```python
from build123d import *

# Parameters (mm, degrees)
BOSS_EXTRUDE1_DEPTH          = 19.05
SKETCH2_W                    = 12.7
SKETCH2_H                    = 9.652
CUT_EXTRUDE1_DEPTH           = 108.035088344
BOSS_EXTRUDE2_DEPTH          = 3.175
CUT_EXTRUDE12_DEPTH          = 7.9375
F_1_2_0_375_DIAMETER_HOLE1_D = 9.525
F_1_2_0_375_DIAMETER_HOLE2_D = 9.525


with BuildPart() as part:
    # Sketch1 → Boss-Extrude1 (new, symmetric)
    with BuildSketch(Plane.XY):
        with BuildLine():
            Line((0, 36.148070179), (0, 0))
            Line((0, 0), (88.9, 0))
            Line((88.9, 0), (88.9, 19.05))
            Line((88.9, 19.05), (28.593563708, 53.867937227))
            ThreePointArc((28.593563708, 53.867937227), (8.995572876, 53.562269727), (0, 36.148070179))
        make_face()
    extrude(amount=BOSS_EXTRUDE1_DEPTH, both=True)

    # Sketch2 → Cut-Extrude1 (cut, through all)
    with BuildSketch(Plane(origin=(88.9, 0, 0), x_dir=(0, 0, -1), z_dir=(1, 0, 0))):
        with Locations((0, 4.826)):
            Rectangle(SKETCH2_W, SKETCH2_H)
    extrude(amount=-CUT_EXTRUDE1_DEPTH, mode=Mode.SUBTRACT)

    # Sketch3 → Boss-Extrude2 (add, symmetric)
    with BuildSketch(Plane.XY.offset(12.7)):
        Polygon((88.9, 28.728699913), (61.669909488, 44.45), (44.905909488, 44.45), (88.9, 19.05), align=None)
    extrude(amount=BOSS_EXTRUDE2_DEPTH, both=True)

    # Sketch17 → Cut-Extrude12 (cut, symmetric)
    with BuildSketch(Plane.XY):
        Polygon((0, 25.4), (33.782, 25.4), (51.929375197, 56.832175865), (0, 56.832175865), align=None)
    extrude(amount=CUT_EXTRUDE12_DEPTH, both=True, mode=Mode.SUBTRACT)

    # 1/2 (0.375) Diameter Hole1 (through all)
    with Locations(Plane(origin=(30.473891971, 52.782329198, 0), x_dir=(0.8660254037844419, -0.4999999999999945, 0), z_dir=(0.49999999999999445, 0.8660254037844418, 0))):
        with Locations((42.064658396, 0)):
            Hole(F_1_2_0_375_DIAMETER_HOLE1_D / 2)

    # 1/2 (0.375) Diameter Hole2 (through all)
    with Locations(Plane.XY.offset(19.05)):
        with Locations((19.05, 37.338)):
            Hole(F_1_2_0_375_DIAMETER_HOLE2_D / 2)


solid = part.part
```
Source: CAD feature listing. Evaluate the final solid. Frame: model axes, mm. A direction names the side the tool comes from. Coordinates: 2 decimals unless noted, no trailing zeros. Write each loop counter-clockwise with the first axis right and the second up, starting at its lowest first coordinate (ties: lowest second). Pieces come first, ordered by that corner, then holes. Notation, with made-up numbers: (-27.5, -18) - (7.5, -18) arc R23 ccw to (7.5, 3) - close; hole circle Ø5 at (-3.75, 25.5). An arc over 180 degrees is marked (long way). Answer as a JSON object with one key per item and string values.
Q1. Set-up query: faces 4 (the cylindrical face through (16.49, 41.354, -13.572)), 5 (the flat face through (45, 5, -6.35)), 6 (the flat face through (53, 44.45, 13)), 7 (the flat face through (72, 35, 15.875)). Return all of +Z, -Z, +X, -X, +Y, -Y with unobstructed straight access to the full face (end or side cutting, diameter ignored); none if empty.
Ans:
{"face 4": "+Z, -Z", "face 5": "+X, -X, -Y", "face 6": "+Z, -Z, +X, +Y", "face 7": "+Z, +X, +Y"}
Q2. First-contact query: pin 1 Ø5 at (x, z) = (53.5, 13) entering from +Y; pin 2 Ø1 at (y, z) = (30.5, 1) entering from -X; pin 3 Ø1.5 at (y, z) = (31.5, 0.5) entering from -X. Flat tips, straight axial feed; report the tip coordinate or a pass-through.
Ans:
{"pin 1": "stops at y = 44.45", "pin 2": "stops at x = 36.44", "pin 3": "stops at x = 36.87"}
Q3. Draft query along Z for faces 1 (the flat face through (34, 22, 19.05)), 2 (the flat face through (59.169, 36.215, 0.267)), 3 (the flat face through (45, 9.652, 0)). Return one class per face: released by +Z, released by -Z, zero draft, split by the parting line, or undercut.
Ans:
{"face 1": "released by +Z", "face 2": "zero draft", "face 3": "undercut"}
Q4. Section query A-A, the plane x = 19.05. Output: boundary loops of the cut face in (y, z).
Ans:
{"outline": "(0, -19.05) - (32.58, -19.05) - (32.58, -7.94) - (25.4, -7.94) - (25.4, 7.94) - (32.58, 7.94) - (32.58, 19.05) - (0, 19.05) - (0, 6.35) - (9.65, 6.35) - (9.65, -6.35) - (0, -6.35) - close; (42.1, -19.05) - (56.43, -19.05) - (56.43, -7.94) - (42.1, -7.94) - close; (42.1, 7.94) - (56.43, 7.94) - (56.43, 19.05) - (42.1, 19.05) - close"}
Q5. Material intervals for line 1 (Z direction, x = 25.5, y = 7); line 2 (Z direction, x = 59, y = 18); line 3 (Y direction, x = 19.05, z = 15.5), sorted ascending. Write a range as [from, to].
Ans:
{"line 1": "z = [-19.05, -6.35], [6.35, 19.05]", "line 2": "z = [-19.05, -4.76], [4.76, 19.05]", "line 3": "y = [0, 32.58], [42.1, 56.43]"}
Q6. Section query D-D, the plane x = 47.5. Output: boundary loops of the cut face in (y, z) (3 decimals), plus the area to 3 significant figures.
Ans:
{"outline": "(0, -19.05) - (42.952, -19.05) - (42.952, 9.525) - (44.45, 9.525) - (44.45, 15.875) - (42.952, 15.875) - (42.952, 19.05) - (0, 19.05) - (0, 6.35) - (9.652, 6.35) - (9.652, -6.35) - (0, -6.35) - close", "area": "1,520 mm2"}
Q7. Section query B-B, the plane y = 7. Output: boundary loops of the cut face in (x, z), plus the area to 3 significant figures.
Ans:
{"outline": "(0, -19.05) - (88.9, -19.05) - (88.9, -6.35) - (0, -6.35) - close; (0, 6.35) - (88.9, 6.35) - (88.9, 19.05) - (0, 19.05) - close", "area": "2,260 mm2"}
Q8. Section query C-C, the plane z = -3. Output: boundary loops of the cut face in (x, y), plus the area to 3 significant figures.
Ans:
{"outline": "(0, 9.65) - (49.87, 9.65) - (63.7, 33.6) - (44.81, 44.5) - (33.78, 25.4) - (0, 25.4) - close; (0, 36.15) - (0, 38.53) arc R19.09 ccw to start; (58.42, 9.65) - (88.9, 9.65) - (88.9, 19.05) - (70.11, 29.9) - close", "area": "1,600 mm2"}
